Model file for the job. Use its own axes, mm. Face numbers are marked on the shaded views. Coordinates: 2 decimals unless noted, no trailing zeros. Write each loop counter-clockwise with the first axis right and the second up, starting at its lowest first coordinate (ties: lowest second). Pieces come first, ordered by that corner, then holes.
Q1. Band-saw the part on D-D, the plane y = -1.3. Write the cut outline in (x, z), plus the area to 3 significant figures.
Q2. Band-saw the part on B-B, the plane y = -2.15. Write the cut outline in (x, z), plus the area to 3 significant figures.
Q3. Pin check, flat tips, straight feed: P1, Ø0.5, axis at x = -1.5, z = 14, coming from the -Y side; P2, Ø0.7, axis at y = 1.5, z = 10, coming from the +X side; P3, Ø0.5, axis at x = 1, y = 1, coming from the +Z side. Stop position of each tip, or through.
Q4. Band-saw the part on A-A, the plane z = 9. Write the cut outline in (x, y).
Q5. Band-saw the part on C-C, the plane y = 1.7. Write the cut outline in (x, z), plus the area to 3 significant figures.
Q6. Pull direction X, two halves, no side cores. Call the marked faces 1, 2, 3 and 4: released by +X, released by -X, zero draft, split by the parting line, or undercut.
Q7. Drill centre lines: probe 1 along Z at (x, y) = (1.5, -0.3); probe 2 along Y at (x, z) = (1.55, 13); probe 3 along Z at (x, y) = (1.6, -1.95). Where is each one in solid material? Low to high.
from build123d import *

# Parameters (mm, degrees)
SKETCH1_R           = 2
BOSS_EXTRUDE1_DEPTH = 13.5
SKETCH2_R           = 1.2
CUT_EXTRUDE1_DEPTH  = 14.793114224
SKETCH3_W           = 0.8
SKETCH3_H           = 6.59267807
SKETCH3_W_2         = 7.006923124
SKETCH3_H_2         = 0.8
CUT_EXTRUDE3_DEPTH  = 14.793114224
BOSS_EXTRUDE2_DEPTH = 1
SKETCH5_R           = 3
BOSS_EXTRUDE3_DEPTH = 1


with BuildPart() as part:
    # Sketch1 → Boss-Extrude1 (new body)
    with BuildSketch(Plane.XY):
        Circle(SKETCH1_R)
    extrude(amount=BOSS_EXTRUDE1_DEPTH)

    # Sketch2 → Cut-Extrude1 (cut, through all)
    with BuildSketch(Plane.XY.offset(13.5)):
        Circle(SKETCH2_R)
    extrude(amount=-CUT_EXTRUDE1_DEPTH, mode=Mode.SUBTRACT)

    # Sketch3 → Cut-Extrude3 (cut, through all)
    with BuildSketch(Plane.XY.offset(13.5)):
        Rectangle(SKETCH3_W, SKETCH3_H)
        Rectangle(SKETCH3_W_2, SKETCH3_H_2)
    extrude(amount=-CUT_EXTRUDE3_DEPTH, mode=Mode.SUBTRACT)


with BuildPart() as cut_extrude3_piece_1:
    # of the separate pieces the step leaves, piece 1, a body of its own (cut_extrude3_pieces)
    add(part.part.solids().sort_by_distance((1.959591794, 0.4, 0))[0])



with BuildPart() as cut_extrude3_piece_2:
    # of the separate pieces the step leaves, piece 2, a body of its own (cut_extrude3_pieces)
    add(part.part.solids().sort_by_distance((0.4, -1.959591794, 0))[0])



with BuildPart() as cut_extrude3_piece_3:
    # of the separate pieces the step leaves, piece 3, a body of its own (cut_extrude3_pieces)
    add(part.part.solids().sort_by_distance((-1.959591794, -0.4, 0))[0])


with BuildPart() as cut_extrude3_piece_4:
    # of the separate pieces the step leaves, piece 4, a body of its own (cut_extrude3_pieces)
    add(part.part.solids().sort_by_distance((-0.4, 1.959591794, 0))[0])


with BuildPart() as cut_extrude3_piece_2_1:
    add(cut_extrude3_piece_2.part)

    add(cut_extrude3_piece_4.part)  # Boss-Extrude2 merges Cut-Extrude3 piece 4
    # Sketch4 → Boss-Extrude2 (add)
    with BuildSketch(Plane.XY.offset(13.5)):
        with BuildLine():
            Line((-2.297825059, 0.1), (-1.13137085, 0.1))
            Line((-1.13137085, 0.1), (-1.13137085, 0.4))
            ThreePointArc((-1.13137085, 0.4), (-0.848528137, 0.848528137), (-0.4, 1.13137085))
            Line((-0.4, 1.13137085), (-0.1, 1.13137085))
            Line((-0.1, 1.13137085), (-0.1, 2.297825059))
            ThreePointArc((-0.1, 2.297825059), (-1.626345597, 1.626345597), (-2.297825059, 0.1))
        make_face()
        with BuildLine():
            Line((0.1, -1.13137085), (0.1, -2.297825059))
            ThreePointArc((0.1, -2.297825059), (1.626345597, -1.626345597), (2.297825059, -0.1))
            Line((2.297825059, -0.1), (1.13137085, -0.1))
            Line((1.13137085, -0.1), (1.13137085, -0.4))
            ThreePointArc((1.13137085, -0.4), (0.848528137, -0.848528137), (0.4, -1.13137085))
            Line((0.4, -1.13137085), (0.1, -1.13137085))
        make_face()
    extrude(amount=BOSS_EXTRUDE2_DEPTH)


with BuildPart() as cut_extrude3_piece_1_1:
    add(cut_extrude3_piece_1.part)

    add(cut_extrude3_piece_2_1.part)  # Boss-Extrude3 merges Cut-Extrude3 piece 2

    add(cut_extrude3_piece_3.part)  # Boss-Extrude3 merges Cut-Extrude3 piece 3
    # Sketch5 → Boss-Extrude3 (add)
    with BuildSketch(Plane(origin=(0, 0, 0), x_dir=(-1, 0, 0), z_dir=(0, 0, -1))):
        Circle(SKETCH5_R)
    extrude(amount=BOSS_EXTRUDE3_DEPTH)


solid = cut_extrude3_piece_1_1.part
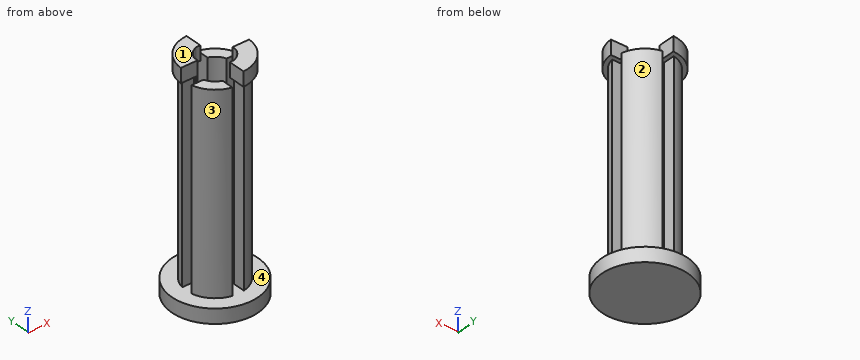
Answer sheet:
1. outline: (-2.7, -1) - (2.7, -1) - (2.7, 0) - (1.52, 0) - (1.52, 13.5) - (1.9, 13.5) - (1.9, 14.5) - (0.1, 14.5) - (0.1, 13.5) - (0.4, 13.5) - (0.4, 0) - (-0.4, 0) - (-0.4, 13.5) - (-1.52, 13.5) - (-1.52, 0) - (-2.7, 0) - close
1. area: 37.4 mm2
2. outline: (-2.09, -1) - (2.09, -1) - (2.09, 0) - (-2.09, 0) - close; (0.1, 13.5) - (0.82, 13.5) - (0.82, 14.5) - (0.1, 14.5) - close
2. area: 4.90 mm2
3. P1: stops at y = 0.1
3. P2: stops at x = 1.64
3. P3: stops at z = 13.5
4. outline: (-1.96, -0.4) arc R2 ccw to (-0.4, -1.96) - (-0.4, -1.13) arc R1.2 cw to (-1.13, -0.4) - close; (-1.96, 0.4) - (-1.13, 0.4) arc R1.2 cw to (-0.4, 1.13) - (-0.4, 1.96) arc R2 ccw to start; (0.4, -1.96) arc R2 ccw to (1.96, -0.4) - (1.13, -0.4) arc R1.2 cw to (0.4, -1.13) - close; (0.4, 1.13) arc R1.2 cw to (1.13, 0.4) - (1.96, 0.4) arc R2 ccw to (0.4, 1.96) - close
5. outline: (-2.47, -1) - (2.47, -1) - (2.47, 0) - (1.05, 0) - (1.05, 13.5) - (0.4, 13.5) - (0.4, 0) - (-0.4, 0) - (-0.4, 13.5) - (-0.1, 13.5) - (-0.1, 14.5) - (-1.55, 14.5) - (-1.55, 13.5) - (-1.05, 13.5) - (-1.05, 0) - (-2.47, 0) - close
5. area: 24.0 mm2
6. face 1: zero draft
6. face 2: released by +X
6. face 3: released by -X
6. face 4: undercut
7. probe 1: z = -1 to 0, 13.5 to 14.5
7. probe 2: y = -1.26 to -0.4, 0.4 to 1.26
7. probe 3: z = -1 to 0
